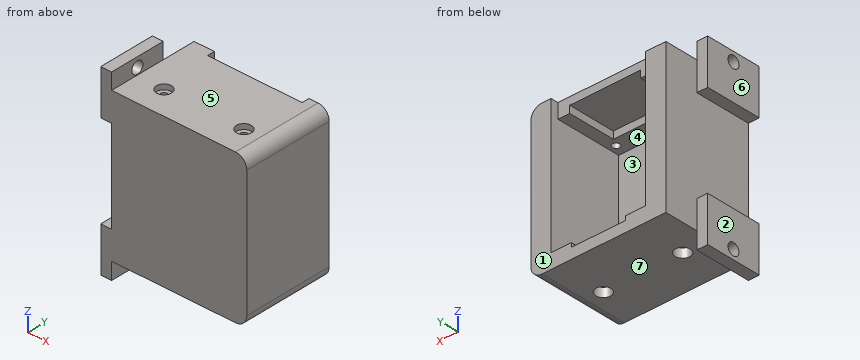
from build123d import *

# Parameters (mm, degrees)
SKETCH_3_W           = 36
SKETCH_3_H           = 50
EXTRUDE_1_DEPTH      = 24
SKETCH_4_W           = 24.8
SKETCH_4_H           = 31.8
CUT_EXTRUDE_1_DEPTH  = 19.7
SKETCH_5_W           = 14
SKETCH_5_H           = 2.2
CUT_EXTRUDE_3_DEPTH  = 19.7
SKETCH_6_W           = 18.5
SKETCH_6_H           = 3.8
CUT_EXTRUDE_4_DEPTH  = 14.7
SKETCH_7_W           = 24.8
SKETCH_7_H           = 24.280407208
CUT_EXTRUDE_5_DEPTH  = 2
SKETCH_8_R           = 2
CUT_EXTRUDE_6_DEPTH  = 6.4
SKETCH_9_R           = 1
CUT_EXTRUDE_7_DEPTH  = 6.4
SKETCH_10_R          = 2
CUT_EXTRUDE_8_DEPTH  = 7.4
SKETCH_11_R          = 1
CUT_EXTRUDE_9_DEPTH  = 7.4
SKETCH_14_W          = 47.693248889
SKETCH_14_H          = 41.94352182
CUT_EXTRUDE_12_DEPTH = 4
SKETCH_16_W          = 69.166934332
SKETCH_16_H          = 39.422219991
CUT_EXTRUDE_13_DEPTH = 5
CUT_EXTRUDE_17_DEPTH = 19.7
SKETCH_19_W          = 18.9
SKETCH_19_H          = 2.1
CUT_EXTRUDE_18_DEPTH = 12.7
SKETCH_21_W          = 12
SKETCH_21_H          = 15
EXTRUDE_2_DEPTH      = 2.9
SKETCH_24_W          = 40.92959711
SKETCH_24_H          = 30.072359406
CUT_EXTRUDE_20_DEPTH = 1
SKETCH_23_R          = 1.6
CUT_EXTRUDE_21_DEPTH = 10
SKETCH_25_W          = 25.2
SKETCH_25_H          = 37.099500986
CUT_EXTRUDE_22_DEPTH = 2
FILLET_1_R           = 3


with BuildPart() as part:
    # 草图3 → 凸台-拉伸1 (new body)
    with BuildSketch(Plane(origin=(0, 0, 0), x_dir=(1, 0, 0), z_dir=(0, 1, 0))):
        Rectangle(SKETCH_3_W, SKETCH_3_H)
    extrude(amount=EXTRUDE_1_DEPTH)

    # 草图4 → 切除-拉伸1 (cut)
    with BuildSketch(Plane(origin=(0, 24, 0), x_dir=(1, 0, 0), z_dir=(0, 1, 0))):
        Rectangle(SKETCH_4_W, SKETCH_4_H)
    extrude(amount=-CUT_EXTRUDE_1_DEPTH, mode=Mode.SUBTRACT)

    # 草图5 → 切除-拉伸3 (cut)
    with BuildSketch(Plane(origin=(0, 24, 0), x_dir=(1, 0, 0), z_dir=(0, 1, 0))):
        with Locations((0, 15.9)):
            Rectangle(SKETCH_5_W, SKETCH_5_H)
    extrude(amount=-CUT_EXTRUDE_3_DEPTH, mode=Mode.SUBTRACT)

    # 草图6 → 切除-拉伸4 (cut)
    with BuildSketch(Plane(origin=(0, 24, 0), x_dir=(1, 0, 0), z_dir=(0, 1, 0))):
        with Locations((0, -15.9)):
            Rectangle(SKETCH_6_W, SKETCH_6_H)
    extrude(amount=-CUT_EXTRUDE_4_DEPTH, mode=Mode.SUBTRACT)

    # 草图7 → 切除-拉伸5 (cut)
    with BuildSketch(Plane(origin=(0, 24, 0), x_dir=(1, 0, 0), z_dir=(0, 1, 0))):
        with Locations((0, -25)):
            Rectangle(SKETCH_7_W, SKETCH_7_H)
    extrude(amount=-CUT_EXTRUDE_5_DEPTH, mode=Mode.SUBTRACT)

    # 草图8 → 切除-拉伸6 (cut)
    with BuildSketch(Plane.XY.offset(25)):
        with Locations((10.65, 7.2)):
            Circle(SKETCH_8_R)
        with Locations((-10.65, 7.2)):
            Circle(SKETCH_8_R)
    extrude(amount=-CUT_EXTRUDE_6_DEPTH, mode=Mode.SUBTRACT)

    # 草图9 → 切除-拉伸7 (cut)
    with BuildSketch(Plane.XY.offset(18.6)):
        with Locations((10.65, 7.2)):
            Circle(SKETCH_9_R)
        with Locations((-10.65, 7.2)):
            Circle(SKETCH_9_R)
    extrude(amount=-CUT_EXTRUDE_7_DEPTH, mode=Mode.SUBTRACT)

    # 草图10 → 切除-拉伸8 (cut)
    with BuildSketch(Plane(origin=(0, 0, -25), x_dir=(-1, 0, 0), z_dir=(0, 0, -1))):
        with Locations((-10.565, 11)):
            Circle(SKETCH_10_R)
        with Locations((10.56, 11)):
            Circle(SKETCH_10_R)
    extrude(amount=-CUT_EXTRUDE_8_DEPTH, mode=Mode.SUBTRACT)

    # 草图11 → 切除-拉伸9 (cut)
    with BuildSketch(Plane(origin=(0, 0, -17.6), x_dir=(-1, 0, 0), z_dir=(0, 0, -1))):
        with Locations((10.56, 11)):
            Circle(SKETCH_11_R)
        with Locations((-10.565, 11)):
            Circle(SKETCH_11_R)
    extrude(amount=-CUT_EXTRUDE_9_DEPTH, mode=Mode.SUBTRACT)

    # 草图14 → 切除-拉伸12 (cut)
    with BuildSketch(Plane.XY.offset(25)):
        with Locations((-2.653720185, 12.393348568)):
            Rectangle(SKETCH_14_W, SKETCH_14_H)
    extrude(amount=-CUT_EXTRUDE_12_DEPTH, mode=Mode.SUBTRACT)

    # 草图16 → 切除-拉伸13 (cut)
    with BuildSketch(Plane(origin=(0, 0, -25), x_dir=(-1, 0, 0), z_dir=(0, 0, -1))):
        with Locations((0.858826259, 12.588310345)):
            Rectangle(SKETCH_16_W, SKETCH_16_H)
    extrude(amount=-CUT_EXTRUDE_13_DEPTH, mode=Mode.SUBTRACT)

    # 草图18 → 切除-拉伸17 (cut)
    with BuildSketch(Plane(origin=(0, 24, 0), x_dir=(1, 0, 0), z_dir=(0, 1, 0))):
        Polygon((-12.6, -16.1), (12.6, -16.1), (12.6, 16.1), (7.2, 16.1), (7.2, 17.2), (-7.2, 17.2), (-7.2, 16.1), (-12.6, 16.1), align=None)
    extrude(amount=-CUT_EXTRUDE_17_DEPTH, mode=Mode.SUBTRACT)

    # 草图19 → 切除-拉伸18 (cut)
    with BuildSketch(Plane(origin=(0, 22, 0), x_dir=(1, 0, 0), z_dir=(0, 1, 0))):
        with Locations((0, -16.95)):
            Rectangle(SKETCH_19_W, SKETCH_19_H)
    extrude(amount=-CUT_EXTRUDE_18_DEPTH, mode=Mode.SUBTRACT)

    # 草图21 → 凸台-拉伸2 (add)
    with BuildSketch(Plane.ZY.offset(18)):
        with Locations((-18.5, 7.5)):
            Rectangle(SKETCH_21_W, SKETCH_21_H)
        with Locations((18.3, 7.5)):
            Rectangle(SKETCH_21_W, SKETCH_21_H)
    extrude(amount=EXTRUDE_2_DEPTH)

    # 草图24 → 切除-拉伸20 (cut)
    with BuildSketch(Plane.XY.offset(21)):
        with Locations((2.464798555, 15.036179703)):
            Rectangle(SKETCH_24_W, SKETCH_24_H)
    extrude(amount=-CUT_EXTRUDE_20_DEPTH, mode=Mode.SUBTRACT)

    # 草图23 → 切除-拉伸21 (cut)
    with BuildSketch(Plane.ZY.offset(20.9)):
        with Locations((-22, 7.5)):
            Circle(SKETCH_23_R)
        with Locations((21.8, 7.5)):
            Circle(SKETCH_23_R)
    extrude(amount=-CUT_EXTRUDE_21_DEPTH, mode=Mode.SUBTRACT)

    # 草图25 → 切除-拉伸22 (cut)
    with BuildSketch(Plane(origin=(0, 24, 0), x_dir=(1, 0, 0), z_dir=(0, 1, 0))):
        with Locations((0, -2.449750493)):
            Rectangle(SKETCH_25_W, SKETCH_25_H)
    extrude(amount=-CUT_EXTRUDE_22_DEPTH, mode=Mode.SUBTRACT)

    # 圆角1
    fillet_1_edges = [part.edges().sort_by_distance(p)[0] for p in [
        (18, 12, -20),
        (18, 12, 20),
    ]]
    fillet(fillet_1_edges, radius=FILLET_1_R)


solid = part.part
Could you check a few things on this model? Use its own coordinates, in mm. Face numbers are marked on the shaded views. A direction names the side the tool comes from. Coordinates: 2 decimals unless noted, no trailing zeros. Loops run counter-clockwise (first coordinate to the right, second up) from the corner with the lowest first, then second, coordinate; pieces in that order, holes last.
1. Imagine slicing it at B-B (x = -10.56). Please give me the cut outline in (y, z).
2. Imagine slicing it at D-D (x = 6). Please give me the cut outline in (y, z), and give its area (3 significant figures).
3. Imagine slicing it at A-A (z = -22). Please give me the cut outline in (x, y), and give its area (3 significant figures).
4. For P1, Ø8, axis at x = -4, y = 7.5, coming from the -Z side; P2, Ø2, axis at x = 11.5, z = 2, coming from the +Y side; P3, Ø3, axis at y = 6.5, z = -3.5, coming from the -X side, each with a flat end and sliding along its axis, tell me the tip position at first contact or that it passes through.
5. I need wall thicknesses on L1, parallel to Y at x = -19.25, z = -22; L2, parallel to X at y = 7.75, z = -10.5; L3, parallel to Z at x = -9, y = 8.5. Which ranges of each line are inside material? Lowest first, please.
6. Imagine slicing it at C-C (y = 2.5). Please give me the cut outline in (x, z).
7. We'd pull the mould along X, two halves only. Please class the marked faces 1, 2 and 3: released by +X, released by -X, zero draft, split by the parting line, or undercut.
8. For the marked faces 4, 5, 6 and 7, which set-ups out of +Z, -Z, +X, -X, +Y, -Y let a thin tool reach every point of the face, with its end or its side?
Computed values:
1. outline: (0, -20) - (9, -20) - (9, -17.6) - (10, -17.6) - (10, -16.1) - (4.3, -16.1) - (4.3, 16.1) - (6.2, 16.1) - (6.2, 18.6) - (5.2, 18.6) - (5.2, 20) - (0, 20) - close; (8.2, 16.1) - (22, 16.1) - (22, 20) - (9.2, 20) - (9.2, 18.6) - (8.2, 18.6) - close; (12, -17.6) - (13, -17.6) - (13, -20) - (24, -20) - (24, -16.1) - (12, -16.1) - close
2. outline: (0, -20) - (24, -20) - (24, -17.2) - (4.3, -17.2) - (4.3, 16.1) - (9.3, 16.1) - (9.3, 18) - (22, 18) - (22, 20) - (0, 20) - close
2. area: 272 mm2
3. outline: (-20.9, 0) - (-18, 0) - (-18, 5.9) - (-20.9, 5.9) - close; (-20.9, 9.1) - (-18, 9.1) - (-18, 15) - (-20.9, 15) - close
3. area: 34.2 mm2
4. P1: stops at z = -20
4. P2: stops at y = 4.3
4. P3: stops at x = -18
5. L1: y = 0 to 5.9, 9.1 to 15
5. L2: x = -18 to -12.6, 12.6 to 18
5. L3: z = -20 to -16.1, 16.1 to 20
6. outline: (-20.9, -24.5) - (-18, -24.5) - (-18, -20) - (15, -20) arc R3 ccw to (18, -17) - (18, 17) arc R3 ccw to (15, 20) - (-18, 20) - (-18, 24.3) - (-20.9, 24.3) - (-20.9, 12.3) - (-18, 12.3) - (-18, -12.5) - (-20.9, -12.5) - close
7. face 1: zero draft
7. face 2: released by -X
7. face 3: undercut
8. face 4: +Y
8. face 5: +Z, +X, +Y, -Y
8. face 6: +Z, -Z, -X, +Y, -Y
8. face 7: -Z, +X, +Y, -Y
